For this review, take the finished solid that the model builds, in its own axes (mm). Round coordinates to 2 decimals unless told otherwise and drop trailing zeros. Order: outer loops, then holes, each group sorted by start corner. A loop starts at its lowest first (then second) coordinate and runs counter-clockwise, first axis right, second up. Notation, with made-up numbers: (-6, 70.25) - (35, 70.25) arc R37 ccw to (35, 107.25) - close; hole circle Ø5 at (82.25, -6.5). An arc over 180 degrees is marked (long way). One line per item, written item: value.
```python
from build123d import *

# Parameters (mm, degrees)
BASE_FLANGE1_DEPTH = 120
CUT_EXTRUDE1_DEPTH = 10


# Sheet-metal steps are written as plain solids
with BuildPart() as part:
    # Sketch1 → Base-Flange1 (new body)
    with BuildSketch(Plane(origin=(0, 0, 0), x_dir=(1, 0, 0), z_dir=(0, 1, 0))):
        with BuildLine():
            Line((122.5, 0), (212.5, 0))
            ThreePointArc((212.5, 0), (262.5, 13.397459622), (299.102540378, 50))
            Line((299.102540378, 50), (296.504464167, 51.5))
            ThreePointArc((296.504464167, 51.5), (261, 15.995535833), (212.5, 3))
            Line((212.5, 3), (122.5, 3))
            Line((122.5, 3), (122.5, 0))
        make_face()
    extrude(amount=BASE_FLANGE1_DEPTH)

    # Sketch6 → Cut-Extrude1 (cut)
    with BuildSketch(Plane.XY):
        Polygon((122.5, 120), (145, 120), (122.5, 0), align=None)
    extrude(amount=-CUT_EXTRUDE1_DEPTH, mode=Mode.SUBTRACT)

    # Sketch12 → Cut-Revolve1 (revolve, cut)
    with BuildSketch(Plane(origin=(25.631243638, 0, -75.648490011), x_dir=(0.8356082783221033, 0, 0.5493257732890113), z_dir=(0.5493257732890113, 0, -0.8356082783221033))):
        with BuildLine():
            Line((202.75, -82), (370.763557892, -82))
            Line((370.763557892, -82), (370.763557892, -132))
            Line((370.763557892, -132), (132.039321881, -132))
            ThreePointArc((132.039321881, -132), (159.448729811, -95.76275643), (202.75, -82))
        make_face()
    revolve(axis=Axis((25.631243638, 0, -75.648490011), (0, -1, 0)), mode=Mode.SUBTRACT)


solid = part.part
```
Item 1: Take a section at D-D (y = 11.5). Write out the cut boundary in (x, z), plus the area to 3 significant figures.
Returned:
outline: (124.66, -3) - (212.5, -3) arc R97 cw to (296.5, -51.5) - (299.1, -50) arc R100 ccw to (212.5, 0) - (124.66, 0) - close
area: 573 mm^2
Item 2: For P1, Ø2, axis at y = 61.5, z = -41, coming from the +X side; P2, Ø6, axis at y = 64, z = -45.5, coming from the +X side; P3, Ø10, axis at x = 176.5, y = 79, coming from the -Z side, all flat-tipped, find the tip position at first contact; note any pin that passes through.
Returned:
P1: x = 293.96
P2: x = 298.22
P3: z = -3
Item 3: The part is to be moulded in two halves that separate along Y. For faces 1 (the flat face through (210, 0, -1)), 2 (the flat face through (168, 45, -3)), 3 (the flat face through (259.5, 82, -14.9)), say which applies: +Y half, -Y half, draft (parallel to the pull), parting line (faces both ways), or undercut.
Returned:
face 1: -Y half
face 2: draft
face 3: +Y half
Item 4: Take a section at C-C (z = -5.5). Write out the cut boundary in (x, y).
Returned:
outline: (234.38, 0) - (245.21, 0) - (245.21, 82) - (234.38, 82) - close
Item 5: Take a section at A-A (y = 30). Write out the cut boundary in (x, z) (3 decimals), plus the area to 3 significant figures.
Returned:
outline: (128.125, -3) - (212.5, -3) arc R97 cw to (296.504, -51.5) - (299.103, -50) arc R100 ccw to (212.5, 0) - (128.125, 0) - close
area: 563 mm^2
Item 6: Wall thickness on line 1 (Z direction, x = 209, y = 78); line 2 (X direction, y = 81.5, z = -37); line 3 (X direction, y = 5.5, z = -38): over which ranges is each line inside the solid? List them lowest first.
Returned:
line 1: -3 to 0
line 2: 286.26 to 290.16
line 3: 287.1 to 290.96
Item 7: Take a section at B-B (x = 140.5). Write out the cut boundary in (y, z), plus the area to 3 significant figures.
Returned:
outline: (0, -3) - (96, -3) - (96, 0) - (0, 0) - close
area: 288 mm^2
